For this review, use the dimensioned drawing (mm, ordinates from the lowest corner) and the shaded views. Coordinates: 2 decimals unless noted, no trailing zeros. Loops run counter-clockwise (first coordinate to the right, second up) from the corner with the lowest first, then second, coordinate; pieces in that order, holes last. Notation, with made-up numbers: (67, -6.5) -> (85, -6.5) arc R22 cw to (85, 23.5) -> close; hole circle Ø7 at (-14, -24.75). An arc over 180 degrees is marked (long way). One line per question, with ' | ' between items. Start each with the question number.
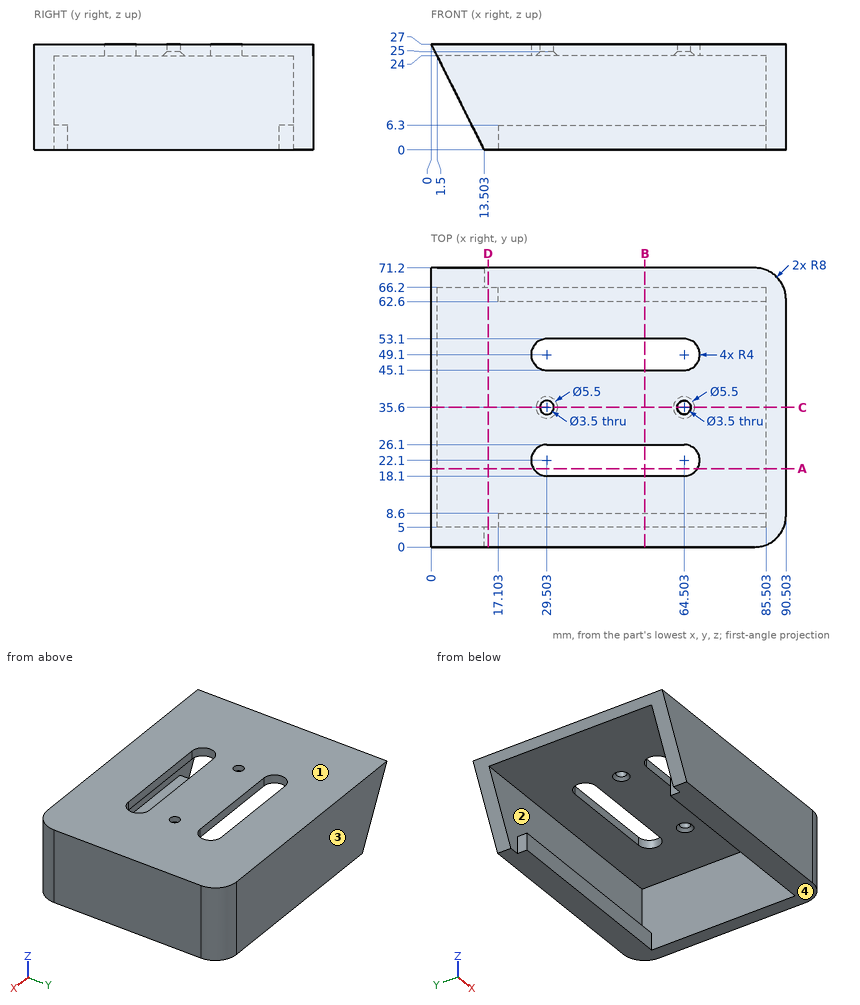
1) Consider section A-A, the plane y = 20. Write out the cut boundary in (x, z).
2) Consider section D-D, the plane x = 14.5. Write out the cut boundary in (y, z).
3) Wall thickness on L1, parallel to Y at x = 62, z = 19.5; L2, parallel to Y at x = 52.5, z = 3.75; L3, parallel to X at y = 14.5, z = 15.25: over which ranges is each line inside the solid? List them lowest first.
4) Consider section C-C, the plane y = 35.6. Write out the cut boundary in (x, z).
5) Insertion check: pin 1 Ø5 at (y, z) = (16.5, 24) entering from -X; pin 2 Ø5 at (y, z) = (43.5, 16.5) entering from -X; pin 3 Ø12 at (x, y) = (65.5, 29.5) entering from -Z. Each pin has a flat end and moves straight along its axis. Give the tip position at first contact, or say it passes through.
6) Consider section B-B, the plane x = 54.5. Write out the cut boundary in (y, z), plus the area to 3 significant figures.
7) Mouldability with a two-part tool opening along Z and no side actions: class the marked faces 1, 2, 3 and 4 as +Z half, -Z half, draft (parallel to the pull), parting line (faces both ways), or undercut.
Filled sheet:
1) outline: (0, 27) -> (1.5, 24) -> (26.1, 24) -> (26.1, 27) -> close; (67.91, 24) -> (85.5, 24) -> (85.5, 0) -> (90.5, 0) -> (90.5, 27) -> (67.91, 27) -> close
2) outline: (0, 0) -> (5, 0) -> (5, 24) -> (66.2, 24) -> (66.2, 0) -> (71.2, 0) -> (71.2, 27) -> (0, 27) -> close
3) L1: 0 to 5, 66.2 to 71.2 | L2: 0 to 8.6, 62.6 to 71.2 | L3: 85.5 to 90.5
4) outline: (0, 27) -> (1.5, 24) -> (26.75, 24) -> (27.75, 25) -> (27.75, 27) -> close; (31.25, 25) -> (32.25, 24) -> (61.75, 24) -> (62.75, 25) -> (62.75, 27) -> (31.25, 27) -> close; (66.25, 25) -> (67.25, 24) -> (85.5, 24) -> (85.5, 0) -> (90.5, 0) -> (90.5, 27) -> (66.25, 27) -> close
5) pin 1: x = 0.25 | pin 2: x = 85.5 | pin 3: z = 24
6) outline: (0, 0) -> (8.6, 0) -> (8.6, 6.3) -> (5, 6.3) -> (5, 24) -> (18.1, 24) -> (18.1, 27) -> (0, 27) -> close; (26.1, 24) -> (45.1, 24) -> (45.1, 27) -> (26.1, 27) -> close; (53.1, 24) -> (66.2, 24) -> (66.2, 6.3) -> (62.6, 6.3) -> (62.6, 0) -> (71.2, 0) -> (71.2, 27) -> (53.1, 27) -> close | area: 451 mm^2
7) face 1: +Z half | face 2: undercut | face 3: draft | face 4: -Z half
